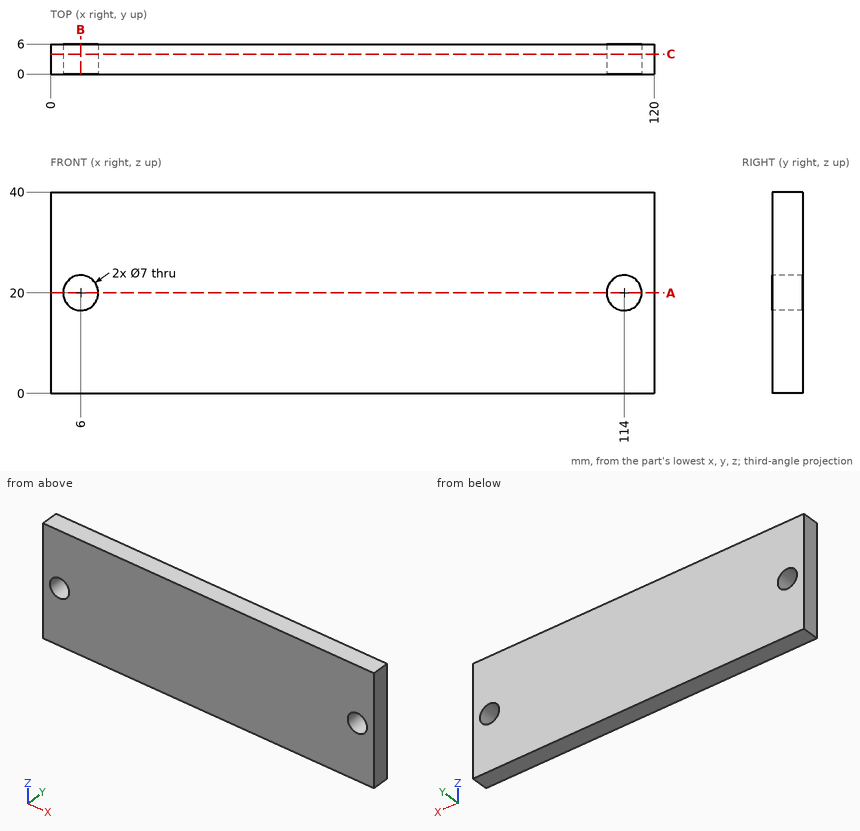
Study the drawing (mm; zero at the part's minimum x, y, z) and answer. Coordinates: 2 decimals unless noted, no trailing zeros. Loops run counter-clockwise (first coordinate to the right, second up) from the corner with the lowest first, then second, coordinate; pieces in that order, holes last. Notation, with made-up numbers: (43.5, -0.5) -> (50.5, -0.5) arc R11 cw to (50.5, 15.5) -> close; hole circle Ø6 at (26.5, -16). An arc over 180 degrees is marked (long way). Answer in a Markdown table with one row per item. Add a question column.
1. The part is cut by section A-A, the plane z = 20. Write down the section's boundary in (x, y).
2. Consider line 1 (X direction, y = 3.5, z = 20); line 2 (Z direction, x = 6, y = 3.75); line 3 (X direction, y = 1, z = 18). Determine where each line is inside the solid, lowest interval first. Write a range as [from, to].
3. A flat-ended cylindrical pin translates along its axis: P1, Ø4, axis at x = 114, z = 20, coming from the -Y side. Find the tip coordinate at first contact, or state that the pin passes through.
4. The part is cut by section B-B, the plane x = 6. Write down the section's boundary in (y, z), then the cut area to 3 significant figures.
5. The part is cut by section C-C, the plane y = 4. Write down the section's boundary in (x, z).
Answer below:
| question | item | result |
|---|---|---|
| 1 | outline | (0, 0) -> (2.5, 0) -> (2.5, 6) -> (0, 6) -> close; (9.5, 0) -> (110.5, 0) -> (110.5, 6) -> (9.5, 6) -> close; (117.5, 0) -> (120, 0) -> (120, 6) -> (117.5, 6) -> close |
| 2 | line 1 | [0, 2.5], [9.5, 110.5], [117.5, 120] |
| 2 | line 2 | [0, 16.5], [23.5, 40] |
| 2 | line 3 | [0, 3.13], [8.87, 111.13], [116.87, 120] |
| 3 | P1 | through |
| 4 | outline | (0, 0) -> (6, 0) -> (6, 16.5) -> (0, 16.5) -> close; (0, 23.5) -> (6, 23.5) -> (6, 40) -> (0, 40) -> close |
| 4 | area | 198 mm2 |
| 5 | outline | (0, 0) -> (120, 0) -> (120, 40) -> (0, 40) -> close; hole circle Ø7 at (6, 20); hole circle Ø7 at (114, 20) |
